Build history of the part. All positions in model axes, mm. Face numbers are marked on the shaded views. Round coordinates to 2 decimals unless told otherwise and drop trailing zeros. Write each loop counter-clockwise with the first axis right and the second up, starting at its lowest first coordinate (ties: lowest second). Pieces come first, ordered by that corner, then holes.
Item 1: Drop flat-ended pins along their axis: pin 1 Ø5 at (x, z) = (-0.5, 2.5) entering from +Y; pin 2 Ø1 at (x, z) = (-19, 1.5) entering from -Y; pin 3 Ø4 at (y, z) = (-10, 6) entering from +X; pin 4 Ø6 at (y, z) = (26.5, 9) entering from +X. Give the stop position or say it passes through.
Item 2: Mould opens along X. For the marked faces 1 and 2 say: +X half, -X half, draft (parallel to the pull), parting line (faces both ways), or undercut.
Item 3: Wall check: probe 1 along X at (y, z) = (59.5, 2.75); probe 2 along Y at (x, z) = (-22, 2); probe 3 along Y at (x, z) = (-17, 0.5). Give the ranges that are in metal, low to high.
Item 4: Band-saw the part on A-A, the plane x = 0. Write the cut outline in (y, z), then the cut area to 3 significant figures.
Item 5: Band-saw the part on B-B, the plane z = 1.5. Write the cut outline in (x, y), then the cut area to 3 significant figures.
```python
from build123d import *

# Parameters (mm, degrees)
F1_DEPTH = 10
F2_W     = 4.8
F2_H     = 4.8
F3_DEPTH = 24
F4_R     = 3


with BuildPart() as f1:
    # F0 (on Top) → F1 (new body)
    with BuildSketch(Plane.XY):
        with BuildLine():
            Line((-30, 0), (30, 0))
            Line((30, 0), (30, 60))
            ThreePointArc((30, 60), (0, 90), (-30, 60))
            Line((-30, 60), (-30, 0))
        make_face()
    extrude(amount=F1_DEPTH)

    # F2 (on face) → F3 (join)
    with BuildSketch(Plane.XZ):
        with Locations((-25, 5)):
            Rectangle(F2_W, F2_H)
        with Locations((-12.5, 5)):
            Rectangle(F2_W, F2_H)
        with Locations((0, 5)):
            Rectangle(F2_W, F2_H)
        with Locations((12.5, 5)):
            Rectangle(F2_W, F2_H)
        with Locations((25, 5)):
            Rectangle(F2_W, F2_H)
    extrude(amount=F3_DEPTH)

    # F4
    f4_edges = [f1.edges().sort_by_distance(p)[0] for p in [
        (30, 30, 10),
        (30, 30, 0),
    ]]
    fillet(f4_edges, radius=F4_R)


solid = f1.part
```
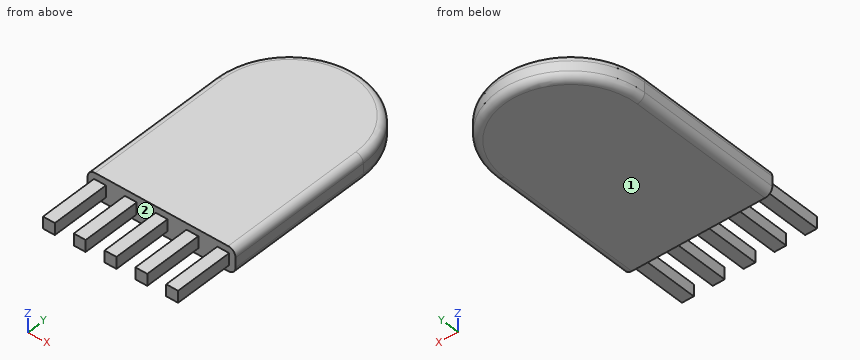
Results:
1. pin 1: stops at y = 90
1. pin 2: stops at y = 0
1. pin 3: stops at x = 27.4
1. pin 4: stops at x = 30
2. face 1: draft
2. face 2: undercut
3. probe 1: x = -29.99 to 29.99
3. probe 2: y = 0 to 80.14
3. probe 3: y = 0 to 83.07
4. outline: (-24, 2.6) - (0, 2.6) - (0, 0) - (87, 0) arc R3 ccw to (90, 3) - (90, 7) arc R3 ccw to (87, 10) - (0, 10) - (0, 7.4) - (-24, 7.4) - close
4. area: 1,010 mm2
5. outline: (-29.6, 0) - (29.6, 0) - (29.6, 60) arc R29.6 ccw to (-29.6, 60) - close
5. area: 4,930 mm2
